from build123d import *

# Parameters (mm, degrees)
SKETCH_W        = 86
SKETCH_H        = 69
PAD_DEPTH       = 50
SKETCH001_W     = 83
SKETCH001_H     = 66
POCKET_DEPTH    = 48.5
SKETCH002_W     = 68
SKETCH002_H     = 50
POCKET001_DEPTH = 5
SKETCH003_W     = 5
SKETCH003_H     = 5
SKETCH003_R     = 1.6
PAD001_DEPTH    = 4
FILLET_R        = 2.25
FILLET001_R     = 2.25
FILLET002_R     = 1.5
SKETCH004_W     = 5
SKETCH004_H     = 5
SKETCH004_R     = 1.6
PAD002_DEPTH    = 48.5
FILLET003_R     = 2.5
FILLET004_R     = 1
FILLET005_R     = 2
CHAMFER_SIZE    = 1.45
SKETCH006_R     = 5
POCKET002_DEPTH = 5
SKETCH007_W     = 9
SKETCH007_H     = 5
POCKET003_DEPTH = 5


with BuildPart() as part:
    # Sketch → Pad (new body)
    with BuildSketch(Plane.XY):
        with Locations((-0.285933, 2.677615)):
            Rectangle(SKETCH_W, SKETCH_H)
    extrude(amount=PAD_DEPTH)

    # Sketch001 (on Face6 of Pad) → Pocket (cut)
    with BuildSketch(Plane.XY.offset(50)):
        with Locations((-0.285933, 2.677615)):
            Rectangle(SKETCH001_W, SKETCH001_H)
    extrude(amount=-POCKET_DEPTH, mode=Mode.SUBTRACT)

    # Sketch002 (on Face11 of Pocket) → Pocket001 (cut)
    with BuildSketch(Plane.XY.offset(1.5)):
        with Locations((-0.285933, 2.677615)):
            Rectangle(SKETCH002_W, SKETCH002_H)
    extrude(amount=-POCKET001_DEPTH, mode=Mode.SUBTRACT)

    # Sketch003 (on Face15 of Pocket001) → Pad001 (join)
    with BuildSketch(Plane.XY.offset(1.5)):
        with Locations((-39.285933, -19.822385)):
            Rectangle(SKETCH003_W, SKETCH003_H)
        with Locations((-39.285933, -19.822385)):
            Circle(SKETCH003_R, mode=Mode.SUBTRACT)
        with Locations((38.714067, 25.177615)):
            Rectangle(SKETCH003_W, SKETCH003_H)
        with Locations((38.714067, 25.177615)):
            Circle(SKETCH003_R, mode=Mode.SUBTRACT)
        with Locations((38.714067, -19.822385)):
            Rectangle(SKETCH003_W, SKETCH003_H)
        with Locations((38.714054, -19.822398)):
            Circle(SKETCH003_R, mode=Mode.SUBTRACT)
        with Locations((-39.285933, 25.177615)):
            Rectangle(SKETCH003_W, SKETCH003_H)
        with Locations((-39.285933, 25.177615)):
            Circle(SKETCH003_R, mode=Mode.SUBTRACT)
    extrude(amount=PAD001_DEPTH)

    # Fillet
    fillet_edges = [part.edges().sort_by_distance(p)[0] for p in [
        (-36.785933, 27.677615, 3.5),
        (-36.785933, 22.677615, 3.5),
    ]]
    fillet(fillet_edges, radius=FILLET_R)

    # Fillet001
    fillet001_edges = [part.edges().sort_by_distance(p)[0] for p in [
        (-36.785933, -17.322385, 3.5),
        (-36.785933, -22.322385, 3.5),
        (36.214067, -17.322385, 3.5),
        (36.214067, -22.322385, 3.5),
        (36.214067, 27.677615, 3.5),
        (36.214067, 22.677615, 3.5),
    ]]
    fillet(fillet001_edges, radius=FILLET001_R)

    # Fillet002
    fillet002_edges = [part.edges().sort_by_distance(p)[0] for p in [
        (41.214067, 22.677615, 3.5),
        (41.214067, 27.677615, 3.5),
        (41.214067, -17.322385, 3.5),
        (41.214067, -22.322385, 3.5),
        (-41.785933, 22.677615, 3.5),
        (-41.785933, 27.677615, 3.5),
        (-41.785933, -17.322385, 3.5),
        (-41.785933, -22.322385, 3.5),
    ]]
    fillet(fillet002_edges, radius=FILLET002_R)

    # Sketch004 (on Face1 of Fillet002) → Pad002 (join)
    with BuildSketch(Plane.XY.offset(1.5)):
        with Locations((-39.285933, -27.822385)):
            Rectangle(SKETCH004_W, SKETCH004_H)
        with Locations((-39.285933, -27.822385)):
            Circle(SKETCH004_R, mode=Mode.SUBTRACT)
        with Locations((-39.285933, 33.177615)):
            Rectangle(SKETCH004_W, SKETCH004_H)
        with Locations((-39.285933, 33.177615)):
            Circle(SKETCH004_R, mode=Mode.SUBTRACT)
        with Locations((38.714067, 33.177615)):
            Rectangle(SKETCH004_W, SKETCH004_H)
        with Locations((38.714067, 33.177615)):
            Circle(SKETCH004_R, mode=Mode.SUBTRACT)
        with Locations((38.714067, -27.822385)):
            Rectangle(SKETCH004_W, SKETCH004_H)
        with Locations((38.714067, -27.822385)):
            Circle(SKETCH004_R, mode=Mode.SUBTRACT)
    extrude(amount=PAD002_DEPTH)

    # Fillet003
    fillet003_edges = [part.edges().sort_by_distance(p)[0] for p in [
        (-36.785933, 30.677615, 25.75),
        (36.214067, 30.677615, 25.75),
        (-36.785933, -25.322385, 25.75),
        (36.214067, -25.322385, 25.75),
    ]]
    fillet(fillet003_edges, radius=FILLET003_R)

    # Fillet004
    fillet004_edges = [part.edges().sort_by_distance(p)[0] for p in [
        (41.214067, -25.322385, 25.75),
        (36.214067, -30.322385, 25.75),
        (41.214067, 30.677615, 25.75),
        (36.214067, 35.677615, 25.75),
        (-41.785933, 30.677615, 25.75),
        (-36.785933, 35.677615, 25.75),
        (-36.785933, -30.322385, 25.75),
        (-41.785933, -25.322385, 25.75),
    ]]
    fillet(fillet004_edges, radius=FILLET004_R)

    # Fillet005
    fillet005_edges = [part.edges().sort_by_distance(p)[0] for p in [
        (-43.285933, 37.177615, 25),
        (42.714067, 37.177615, 25),
        (42.714067, -31.822385, 25),
        (-43.285933, -31.822385, 25),
    ]]
    fillet(fillet005_edges, radius=FILLET005_R)

    # Chamfer
    chamfer_edges = [part.edges().sort_by_distance(p)[0] for p in [
        (-34.285933, 2.677615, 1.5),
        (-0.285933, 27.677615, 1.5),
        (-0.285933, -22.322385, 1.5),
        (33.714067, 2.677615, 1.5),
    ]]
    chamfer(chamfer_edges, length=CHAMFER_SIZE)

    # Sketch006 (on Face13 of Fillet005) → Pocket002 (cut)
    with BuildSketch(Plane.YZ.offset(-41.785933)):
        with Locations((2.677615, 40)):
            Circle(SKETCH006_R)
    extrude(amount=-POCKET002_DEPTH, mode=Mode.SUBTRACT)

    # Sketch007 (on Face25 of Pocket002) → Pocket003 (cut)
    with BuildSketch(Plane(origin=(41.214067, 0, 0), x_dir=(0, -1, 0), z_dir=(-1, 0, 0))):
        with Locations((-2.677615, 47.5)):
            Rectangle(SKETCH007_W, SKETCH007_H)
    extrude(amount=-POCKET003_DEPTH, mode=Mode.SUBTRACT)


solid = part.part
The model under review builds one solid part; all positions refer to its coordinate system, in mm. Give positions to 0.01 mm unless a question says otherwise; leave off trailing zeros. Write each loop counter-clockwise with the first axis right and the second up, starting at its lowest first coordinate (ties: lowest second). Pieces come first, ordered by that corner, then holes.
1. Add section B-B, the plane x = 17. Write out the cut boundary in (y, z).
2. Wall thickness on L1, parallel to X at y = -22.5, z = 34; L2, parallel to Y at x = -17, z = 20; L3, parallel to X at y = 32, z = 27.5: over which ranges is each line inside the solid? List them lowest first.
3. Draft analysis for pull direction Y (two halves, no side actions). For faces 1 (the flat face through (-42, 3, 50)), 2 (the cylindrical face through (-42.716, -31.221, 25.35)), 3 (the flat face through (39, 25, 1.5)), state which applies: +Y half, -Y half, draft (parallel to the pull), parting line (faces both ways), or undercut.
4. For P1, Ø5.5, axis at x = 37.5, y = 25.5, coming from the +Z side; P2, Ø12, axis at x = 29, y = 8, coming from the +Z side, all flat-tipped, find the tip position at first contact; note any pin that passes through.
5. Add section A-A, the plane y = -14.5. Write out the cut boundary in (x, z), plus the area to 3 significant figures.
6. Add section C-C, the plane z = 40. Count the separate pieces of the cut face and the enclosed holes in it, plus the area to 3 significant figures.
Worked answers:
1. outline: (-31.82, 0) - (-22.32, 0) - (-22.32, 0.05) - (-23.77, 1.5) - (-30.32, 1.5) - (-30.32, 50) - (-31.82, 50) - close; (27.68, 0) - (37.18, 0) - (37.18, 50) - (35.68, 50) - (35.68, 1.5) - (29.13, 1.5) - (27.68, 0.05) - close
2. L1: x = -43.29 to -41.79, 41.21 to 42.71
2. L2: y = -31.82 to -30.32, 35.68 to 37.18
2. L3: x = -43.29 to -40.37, -38.2 to -37.08, 36.51 to 37.63, 39.8 to 42.71
3. face 1: draft
3. face 2: -Y half
3. face 3: undercut
4. P1: stops at z = 5.5
4. P2: stops at z = 1.34
5. outline: (-43.29, 0) - (-34.29, 0) - (-34.29, 0.05) - (-35.74, 1.5) - (-41.79, 1.5) - (-41.79, 50) - (-43.29, 50) - close; (33.71, 0) - (42.71, 0) - (42.71, 50) - (41.21, 50) - (41.21, 1.5) - (35.16, 1.5) - (33.71, 0.05) - close
5. area: 170 mm2
6. separate pieces: 1
6. enclosed holes: 4
6. area: 502 mm2
